Autodesk Inventor part; units mm, degrees
ref_plane "YZ Plane" through (0, 0, 0) normal (1, 0, 0) x (0, 1, 0)
ref_plane "XZ Plane" through (0, 0, 0) normal (0, 1, 0) x (-1, 0, 0)
ref_plane "XY Plane" through (0, 0, 0) normal (0, 0, 1) x (1, 0, 0)
sketch "Sketch1" plane through (0, 0, 0) normal (0, 0, 1) x (1, 0, 0)
  line L0 (0, 0) -> (38.1, 0)
  line L1 (38.1, 0) -> (38.1, 6.35)
  line L2 (12.7, 25.4) -> (0, 25.4)
  line L3 (0, 25.4) -> (0, 0)
  line L4 (12.7, 25.4) -> (38.1, 6.35)
  dimension "d2" = 6.35
  dimension "d3" = 12.7
  dimension "d4" = 25.4
  dimension "d5" = 38.1
  dimension "d7" = 27.94
  dimension "d8" = 38.1
extrude "Extrusion1" add sketch "Sketch1" along normal blind 6.35
sketch "Sketch2" plane through (0, 0, 6.35) normal (0, 0, 1) x (1, 0, 0)
  line L0 (0, 0) -> (38.1, 0)
  line L1 (0, 25.4) -> (0, 0)
  line L2 (0, 18.8338) -> (-6.35, 18.8338)
  line L3 (0, 15.1254) -> (-6.35, 15.1254)
  line L4 (15.4827, -6.35) -> (15.4827, 0)
  line L5 (19.1911, -6.35) -> (19.1911, 0)
  line L6 (0, 18.8338) -> (12.7, 18.8338)
  line L7 (13.97, 17.5638) -> (13.97, 16.3954)
  line L8 (12.7, 15.1254) -> (0, 15.1254)
  line L9 (0, 15.1254) -> (0, 18.8338)
  line L10 (19.1911, 0) -> (15.4827, 0)
  line L11 (15.4827, 0) -> (15.4827, 12.7)
  line L12 (16.7527, 13.97) -> (17.9211, 13.97)
  line L13 (19.1911, 12.7) -> (19.1911, 0)
  line L14 (12.7, 18.8338) -> (13.97, 17.5638)
  line L15 (13.97, 16.3954) -> (12.7, 15.1254)
  line L16 (15.4827, 12.7) -> (16.7527, 13.97)
  line L17 (17.9211, 13.97) -> (19.1911, 12.7)
  line L18 (9.144, 20.9166) -> (6.35, 20.9166)
  line L19 (6.35, 20.9166) -> (6.35, 13.0426)
  line L20 (6.35, 13.0426) -> (9.144, 13.0426)
  line L21 (9.144, 13.0426) -> (9.144, 20.9166)
  line L22 (21.2739, 6.35) -> (13.3999, 6.35)
  line L23 (13.3999, 6.35) -> (13.3999, 9.144)
  line L24 (13.3999, 9.144) -> (21.2739, 9.144)
  line L25 (21.2739, 9.144) -> (21.2739, 6.35)
  point P0 (13.97, 15.1254)
  point P1 (13.97, 18.8338)
  point P2 (15.4827, 13.97)
  point P3 (19.1911, 13.97)
  point P4 (19.05, 0)
  dimension "d11" = 13.97
  dimension "d12" = 13.97
  dimension "d13" = 1.27
  dimension "d14" = 1.27
  dimension "d15" = 1.27
  dimension "d16" = 1.27
  dimension "d17" = 1.27
  dimension "d18" = 1.27
  dimension "d19" = 1.27
  dimension "d20" = 1.27
  dimension "d21" = 2.794
  dimension "d22" = 7.874
  dimension "d23" = 6.35
  dimension "d26" = 2.0828
  dimension "d27" = 2.0828
  dimension "d28" = 7.874
  dimension "d29" = 2.794
  dimension "d30" = 2.0828
  dimension "d31" = 6.35
extrude "Extrusion2" cut sketch "Sketch2" against normal through all
equation "\"d26\" = d27"
equation "\"d30\" = d27"
equation "\"d31\" = d23"
properties part number "cornerBraceV01"
Can you work these out from the model? Positions are in its coordinate system, mm. A direction names the side the tool comes from. Give positions to 0.01 mm unless a question says otherwise; leave off trailing zeros. Order: outer loops, then holes, each group sorted by start corner. A loop starts at its lowest first (then second) coordinate and runs counter-clockwise, first axis right, second up. Notation, with made-up numbers: M 18,85 L 31,85 A11 ccw 31,97 Z; hole C 0.5,-10 d1. An arc over 180 degrees is marked long. Write item = value, one per line. Start each with the question number.
Q1. Suppose I cut it at A-A (y = 8). Write out the boundary of the cut face in (x, z), plus the area to 3 significant figures.
Q2. I need wall thicknesses on probe 1 along X at (y, z) = (3.25, 3.25); probe 2 along Y at (x, z) = (8, 1.25); probe 3 along Y at (x, z) = (10, 4.25). Which ranges of each line are inside material? Lowest first, please. Write a range as [from, to].
Q3. For faces 1 (the flat face through (20, 6.35, 3)), 2 (the flat face through (15, 10, 0)), 3 (the flat face through (13.344, 15.769, 3.219)), 4 (the flat face through (0, 22, 3)), 5 (the flat face through (19.191, 11, 3)), which set-ups out of +Z, -Z, +X, -X, +Y, -Y let a thin tool reach every point of the face, with its end or its side?
Q4. Suppose I cut it at D-D (x = 33.5). Write out the boundary of the cut face in (y, z).
Q5. We'd pull the mould along Y, two halves only. Please class faces 6 (the flat face through (18.55, 13.34, 3.22)), 7 (the flat face through (19.191, 3, 3)), 8 (the flat face through (6.35, 20, 3)), 9 (the flat face through (6, 25.4, 3)): pulls with the +Y half, pulls with the -Y half, needs draft (parallel to the pull), parting line crosses it, or undercut.
Q6. Suppose I cut it at B-B (x = 4). Write out the boundary of the cut face in (y, z).
Q7. Will these pins go through, and if not, where does the flat tip stop? pin 1 Ø1.5 at (y, z) = (11.5, 5) entering from +X; pin 2 Ø2.5 at (y, z) = (14, 4.5) entering from +X; pin 3 Ø2.5 at (y, z) = (19.5, 2) entering from +X.
Check result:
q1.outline = M 0,0 L 13.4,0 L 13.4,6.35 L 0,6.35 Z; M 21.27,0 L 35.9,0 L 35.9,6.35 L 21.27,6.35 Z
q1.area = 178 mm2
q2.probe_1 = [0, 15.48], [19.19, 38.1]
q2.probe_2 = [0, 13.04], [20.92, 25.4]
q2.probe_3 = [0, 15.13], [18.83, 25.4]
q3.face_1 = +Z, -Z
q3.face_2 = -Z, +X, -X, +Y, -Y
q3.face_3 = +Z, -Z, -X
q3.face_4 = +Z, -Z, -X, +Y, -Y
q3.face_5 = +Z, -Z, -Y
q4.outline = M 0,0 L 9.8,0 L 9.8,6.35 L 0,6.35 Z
q5.face_6 = pulls with the -Y half
q5.face_7 = needs draft
q5.face_8 = undercut
q5.face_9 = pulls with the +Y half
q6.outline = M 0,0 L 15.13,0 L 15.13,6.35 L 0,6.35 Z; M 18.83,0 L 25.4,0 L 25.4,6.35 L 18.83,6.35 Z
q7.pin_1 = 32.23
q7.pin_2 = 29.57
q7.pin_3 = 22.23
